Build history of the part. All positions in model axes, mm. A direction names the side the tool comes from. Round coordinates to 2 decimals unless told otherwise and drop trailing zeros. Loops run counter-clockwise (first coordinate to the right, second up) from the corner with the lowest first, then second, coordinate; pieces in that order, holes last. Notation, with made-up numbers: (29, 9.25) - (81, 9.25) arc R22 cw to (81, 33.25) - close; hole circle Ø2 at (38, 65). An arc over 180 degrees is marked (long way). Put each result on its own line as item: value. Start each with the question number.
from build123d import *

# Parameters (mm, degrees)
BOSS_EXTRU_1_DEPTH = 3


with BuildPart() as part:
    # Esquisse3 → Boss.-Extru.1 (new body)
    with BuildSketch(Plane(origin=(0, 0, 0), x_dir=(1, 0, 0), z_dir=(0, 1, 0))):
        with BuildLine():
            Line((-65, 21.652023134), (45, 21.652023134))
            ThreePointArc((45, 21.652023134), (55.606601718, 17.258624852), (60, 6.652023134))
            Line((60, 6.652023134), (60, -48.347976866))
            Line((60, -48.347976866), (-80, -48.347976866))
            Line((-80, -48.347976866), (-80, 6.652023134))
            ThreePointArc((-80, 6.652023134), (-75.606601718, 17.258624852), (-65, 21.652023134))
        make_face()
        with BuildLine():
            Line((-45, 1.652023134), (25, 1.652023134))
            ThreePointArc((25, 1.652023134), (40, -13.347976866), (25, -28.347976866))
            Line((25, -28.347976866), (-45, -28.347976866))
            ThreePointArc((-45, -28.347976866), (-60, -13.347976866), (-45, 1.652023134))
        make_face(mode=Mode.SUBTRACT)
    extrude(amount=BOSS_EXTRU_1_DEPTH)


solid = part.part
1) Pull direction Z, two halves, no side cores. Call faces 3 (the face through (55.489, 1.479, -17.375)), 4 (the face through (-59.996, 1.479, 13.678)), 5 (the face through (-9, 0, -3)): pulls with the +Z half, pulls with the -Z half, needs draft (parallel to the pull), parting line crosses it, or undercut.
2) Slice it at C-C, the plane z = 13. Write the cut outline in (x, y), and give its area (3 significant figures).
3) Slice it at A-A, the plane y = 1.65. Write the cut outline in (x, z), and give its area (3 significant figures).
4) Which spindle directions (+Z, -Z, +X, -X, +Y, -Y) get a long thin tool onto all of the face, cutting with end or side? Do faces 1 (the face through (-10, 1, -1.652)), 2 (the face through (-80, 1, 21)). Say none if no direction does.
5) Drill centre lines: line 1 (Z direction, x = -26.5, y = 2.65); line 2 (X direction, y = 1.75, z = 15); line 3 (X direction, y = 2.3, z = 19). Where is each one in solid material? Low to high. Write a range as [from, to].
6) Slice it at B-B, the plane x = -37. Write the cut outline in (y, z).
Taken from the geometry:
1. face 3: pulls with the -Z half
1. face 4: undercut
1. face 5: needs draft
2. outline: (-80, 0) - (-60, 0) - (-60, 3) - (-80, 3) - close; (40, 0) - (60, 0) - (60, 3) - (40, 3) - close
2. area: 120 mm2
3. outline: (-80, -6.65) arc R15 ccw to (-65, -21.65) - (45, -21.65) arc R15 ccw to (60, -6.65) - (60, 48.35) - (-80, 48.35) - close; hole (-45, -1.65) - (25, -1.65) arc R15 ccw to (25, 28.35) - (-45, 28.35) arc R15 ccw to start
3. area: 6,900 mm2
4. face 1: +Y, -Y
4. face 2: +Z, -Z, -X, +Y, -Y
5. line 1: z = [-21.65, -1.65], [28.35, 48.35]
5. line 2: x = [-80, -59.91], [39.91, 60]
5. line 3: x = [-80, -58.89], [38.89, 60]
6. outline: (0, -21.65) - (3, -21.65) - (3, -1.65) - (0, -1.65) - close; (0, 28.35) - (3, 28.35) - (3, 48.35) - (0, 48.35) - close
